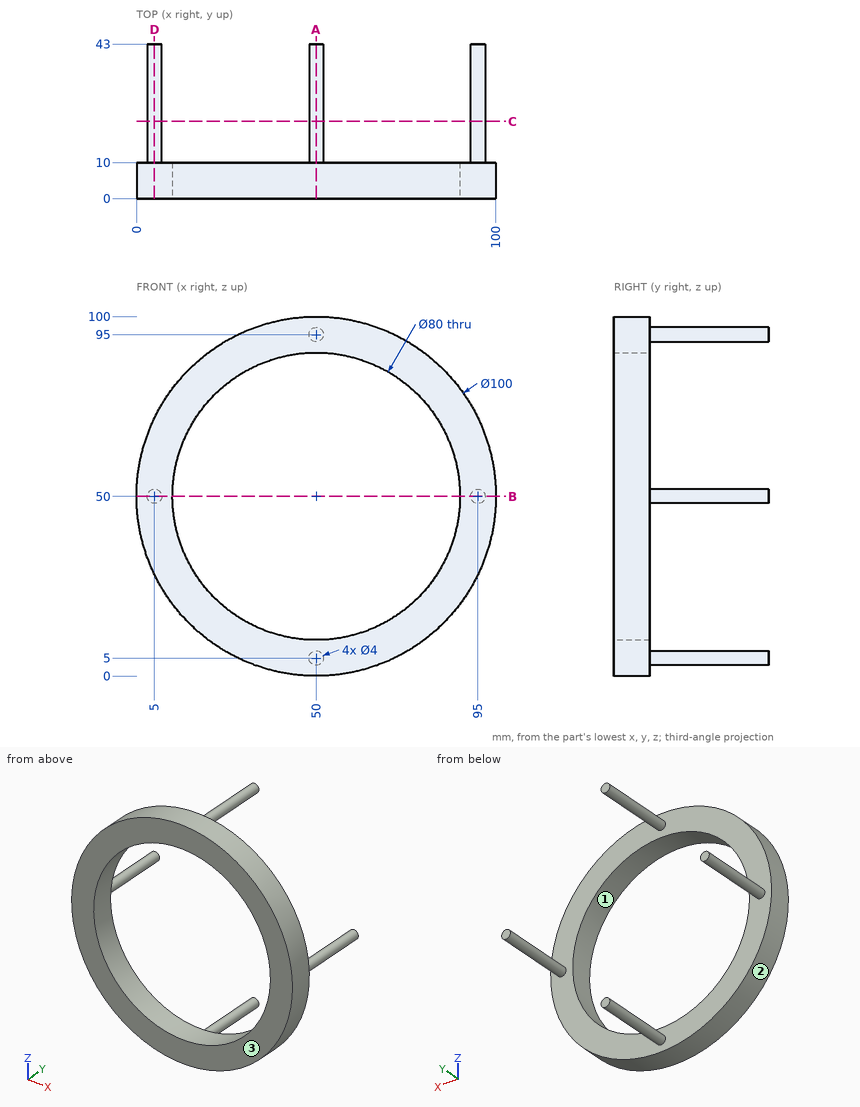
Verification items for this drawing (mm, ordinates from the low corner). Coordinates: 2 decimals unless noted, no trailing zeros. Order: outer loops, then holes, each group sorted by start corner. A loop starts at its lowest first (then second) coordinate and runs counter-clockwise, first axis right, second up.
Q1. Draft check along Z on the marked faces 1, 2 and 3. Enter one of: released by +Z, released by -Z, zero draft, split by the parting line, or undercut.
Reply:
face 1: undercut
face 2: split by the parting line
face 3: zero draft
Q2. Sectioned sample at A-A on x = 50. Record the cut outline in (y, z).
Reply:
outline: (0, 0) - (10, 0) - (10, 3) - (43, 3) - (43, 7) - (10, 7) - (10, 10) - (0, 10) - close; (0, 90) - (10, 90) - (10, 93) - (43, 93) - (43, 97) - (10, 97) - (10, 100) - (0, 100) - close
Q3. Depth check by flat-ended pin: pin 1 Ø8 at (x, y) = (83, 7.5) entering from +Z; pin 2 Ø8 at (x, y) = (34.5, 5) entering from +Z; pin 3 Ø3 at (x, z) = (33.5, 14) entering from +Y. Enter the tip coordinate at first touch or a pass-through.
Reply:
pin 1: stops at z = 90.73
pin 2: stops at z = 98.66
pin 3: stops at y = 10
Q4. Sectioned sample at B-B on z = 50. Record the cut outline in (x, y), and give its area (3 significant figures).
Reply:
outline: (0, 0) - (10, 0) - (10, 10) - (7, 10) - (7, 43) - (3, 43) - (3, 10) - (0, 10) - close; (90, 0) - (100, 0) - (100, 10) - (97, 10) - (97, 43) - (93, 43) - (93, 10) - (90, 10) - close
area: 464 mm2
Q5. Thickness scan on probe 1 along X at (y, z) = (4, 50); probe 2 along X at (y, z) = (2, 47); probe 3 along Y at (x, z) = (78, 9). Record the ranges inside material, lowest first.
Reply:
probe 1: x = 0 to 10, 90 to 100
probe 2: x = 0.09 to 10.11, 89.89 to 99.91
probe 3: y = 0 to 10
Q6. Sectioned sample at C-C on y = 21.5. Record the cut outline in (x, z), and give its area (3 significant figures).
Reply:
outline: circle Ø4 at (5, 50); circle Ø4 at (50, 5); circle Ø4 at (50, 95); circle Ø4 at (95, 50)
area: 50.3 mm2
Q7. Sectioned sample at D-D on x = 5. Record the cut outline in (y, z), and give its area (3 significant figures).
Reply:
outline: (0, 28.21) - (10, 28.21) - (10, 48) - (43, 48) - (43, 52) - (10, 52) - (10, 71.79) - (0, 71.79) - close
area: 568 mm2
